Work out the finished part from the listing and answer in its coordinate system (mm). Face numbers are marked on the shaded views. A direction names the side the tool comes from. Give positions to 0.01 mm unless a question says otherwise; leave off trailing zeros. Write each loop counter-clockwise with the first axis right and the second up, starting at its lowest first coordinate (ties: lowest second). Pieces come first, ordered by that corner, then holes. Notation, with made-up numbers: (-34, 52) - (0, 52) arc R16 cw to (0, 69) - close; hole circle Ø9 at (-17.5, -8.75). An arc over 180 degrees is marked (long way). Write item = value, one per line.
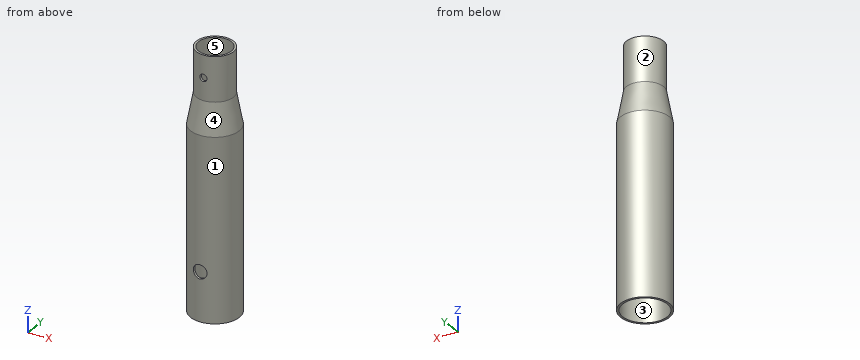
from build123d import *

# Parameters (mm, degrees)
F0_R      = 13.2969
F1_DEPTH  = 31.75
F3_R      = 17.4625
F4_DEPTH  = 130.175
F4_FACE_R = 17.4625
F1_FACE_R = 13.2969
F6_T      = -1.524
F12_D     = 9.92124
F12_DEPTH = 6.35
F12_TIP   = 2.980641204
F13_D     = 5.159375
F13_DEPTH = 6.35
F13_TIP   = 1.5500326281


with BuildPart() as f1:
    # F0 (on Top) → F1 (new body)
    with BuildSketch(Plane.XY):
        Circle(F0_R)
    extrude(amount=-F1_DEPTH)



with BuildPart() as f4:
    # F3 (on offset) → F4 (new body)
    with BuildSketch(Plane.XY.offset(-184.15)):
        Circle(F3_R)
    extrude(amount=F4_DEPTH)


with BuildPart() as f1_1:
    add(f1.part)

    add(f4.part)  # F5 merges F4
    # F4_face (on face) → F5 section 0
    with BuildSketch(Plane.XY.offset(-53.975)):
        Circle(F4_FACE_R)
    # F1_face (on face) → F5 section 1
    with BuildSketch(Plane(origin=(0, 0, -31.75), x_dir=(1, 0, 0), z_dir=(0, 0, -1))):
        Circle(F1_FACE_R)
    loft()

    # F6
    f6_openings = [f1_1.faces().sort_by_distance(p)[0] for p in [
        (0, 0, 0),
        (0, 0, -184.15),
    ]]
    offset(amount=F6_T, openings=f6_openings, kind=Kind.INTERSECTION)

    # F12
    with Locations(Plane.XZ.offset(17.4625)):
        with Locations((0, -149.225)):
            Hole(F12_D / 2, depth=F12_DEPTH)
            with Locations((0, 0, -(F12_DEPTH + F12_TIP / 2))):  # 118° drill point
                Cone(0, F12_D / 2, F12_TIP, mode=Mode.SUBTRACT)

    # F13
    with Locations(Plane.XZ.offset(13.2969)):
        with Locations((0, -15.875)):
            Hole(F13_D / 2, depth=F13_DEPTH)
            with Locations((0, 0, -(F13_DEPTH + F13_TIP / 2))):  # 118° drill point
                Cone(0, F13_D / 2, F13_TIP, mode=Mode.SUBTRACT)


solid = f1_1.part
1. Find section B-B, the plane z = -127. Give the vertices of the cut face in (x, y) (1 decimal), then the cut area to 3 significant figures.
Solution:
outline = circle Ø34.9 at (0, 0); hole circle Ø31.9 at (0, 0)
area = 160 mm^2
2. A tool of negligible diameter and unlimited length cuts with its end or side. For the marked faces 1, 2 and 3, from which of +Z, -Z, +X, -X, +Y, -Y can it reach the whole face along a straight path? Write none if from no direction.
Solution:
face_1 = +Z, -Z
face_2 = +Z
face_3 = -Z
3. Given pin 1 (4 mm diameter, centred on y = 13.5, z = -61, fed in from +X); pin 2 (10 mm diameter, centred on x = 10.5, z = -70.5, fed in from +Y); pin 3 (8 mm diameter, centred on y = -6.5, z = -90, fed in from +X), each flat-ended and moving along its own axis, determine where each tip first touches the part or whether it passes through.
Solution:
pin_1 = 13.14
pin_2 = 16.57
pin_3 = 17.28
4. Find section A-A, the plane x = 0. Give the number of separate pieces and of enclosed holes in the cut face, then the cut area to 3 significant figures.
Solution:
separate_pieces = 4
enclosed_holes = 0
area = 539 mm^2
5. Find section C-C, the plane z = -147. Give the vertices of the cut face in (x, y) (1 decimal).
Solution:
outline = (-4.4, -16.9) - (-4.4, -15.3) arc R15.9 cw (long way) to (4.4, -15.3) - (4.4, -16.9) arc R17.5 ccw (long way) to start
6. For a pull along Y with two mould halves and no side action, classify the marked faces 4 and 5 as pulls with the +Y half, pulls with the -Y half, needs draft (parallel to the pull), parting line crosses it, or undercut.
Solution:
face_4 = parting line crosses it
face_5 = undercut
7. Straight lines are drawn through the part: line 1 (Y direction, x = 0, z = -24.5); line 2 (Y direction, x = 0, z = -15); line 3 (Y direction, x = -6, z = -149.5). For each, find the intervals that lie inside material, in ascending order.
Solution:
line_1 = -13.3 to -11.77, 11.77 to 13.3
line_2 = 11.77 to 13.3
line_3 = -16.4 to -14.77, 14.77 to 16.4
